Part model, mm, in its own coordinate system. A direction names the side the tool comes from. Round coordinates to 2 decimals unless told otherwise and drop trailing zeros. Loops run counter-clockwise (first coordinate to the right, second up) from the corner with the lowest first, then second, coordinate; pieces in that order, holes last. Notation, with made-up numbers: M 28.25,-10.75 L 47.25,-10.75 A33 cw 47.25,28.25 Z; hole C 23.5,-36.5 d3. An arc over 180 degrees is marked long. Put each result on its own line as item: value. Start each with the question number.
```python
from build123d import *

# Parameters (mm, degrees)
SALIENTE_EXTRUIR1_DEPTH      = 5
SALIENTE_EXTRUIR1_DEPTH_BACK = 5
CROQUIS1_W                   = 3
CROQUIS1_H                   = 75
SALIENTE_EXTRUIR3_DEPTH      = 7.5
SALIENTE_EXTRUIR3_DEPTH_BACK = 7.5
CROQUIS1_4_R                 = 3
CROQUIS1_4_R_2               = 1.5
CORTAR_EXTRUIR1_DEPTH        = 2.5
CORTAR_EXTRUIR1_DEPTH_BACK   = 2.5
CROQUIS1_5_R                 = 3
CORTAR_EXTRUIR2_DEPTH        = 10
CORTAR_EXTRUIR2_DEPTH_BACK   = 10
CROQUIS1_6_R                 = 1.5


with BuildPart() as part:
    # Croquis1 → Saliente-Extruir1 (new, two sides: drawn at the far end of the back side and taken through both)
    with BuildSketch(Plane.XY.offset(-SALIENTE_EXTRUIR1_DEPTH_BACK)):
        Rectangle(CROQUIS1_W, CROQUIS1_H)
    extrude(amount=SALIENTE_EXTRUIR1_DEPTH + SALIENTE_EXTRUIR1_DEPTH_BACK)

    # Croquis1_4 → Saliente-Extruir3 (add, two sides: drawn at the far end of the back side and taken through both)
    # profile 1 of 2: a face of its own
    with BuildSketch(Plane.XY.offset(-SALIENTE_EXTRUIR3_DEPTH_BACK)):
        with Locations((0, 37.5)):
            Circle(CROQUIS1_4_R)
        with Locations((0, 37.5)):
            Circle(CROQUIS1_4_R_2, mode=Mode.SUBTRACT)
    # profile 2 of 2: a face of its own
    with BuildSketch(Plane.XY.offset(-SALIENTE_EXTRUIR3_DEPTH_BACK)):
        with Locations((0, -37.5)):
            Circle(CROQUIS1_4_R)
        with Locations((0, -37.5)):
            Circle(CROQUIS1_4_R_2, mode=Mode.SUBTRACT)
    extrude(amount=SALIENTE_EXTRUIR3_DEPTH + SALIENTE_EXTRUIR3_DEPTH_BACK)

    # Croquis1_5 → Cortar-Extruir1 (cut, two sides: drawn at the far end of the back side and taken through both)
    with BuildSketch(Plane.XY.offset(-CORTAR_EXTRUIR1_DEPTH_BACK)):
        with Locations((0, 37.5)):
            Circle(CROQUIS1_5_R)
        with Locations((0, -37.5)):
            Circle(CROQUIS1_5_R)
    extrude(amount=CORTAR_EXTRUIR1_DEPTH + CORTAR_EXTRUIR1_DEPTH_BACK, mode=Mode.SUBTRACT)

    # Croquis1_6 → Cortar-Extruir2 (cut, two sides: drawn at the far end of the back side and taken through both)
    with BuildSketch(Plane.XY.offset(-CORTAR_EXTRUIR2_DEPTH_BACK)):
        with Locations((0, 37.5)):
            Circle(CROQUIS1_6_R)
        with Locations((0, -37.5)):
            Circle(CROQUIS1_6_R)
    extrude(amount=CORTAR_EXTRUIR2_DEPTH + CORTAR_EXTRUIR2_DEPTH_BACK, mode=Mode.SUBTRACT)

    # Croquis1_11 → Cortar-Revoluci_n2 (revolve, cut)
    with BuildSketch(Plane.XY):
        with BuildLine():
            ThreePointArc((-3, -37.5), (0, -40.5), (3, -37.5))
            Line((3, -37.5), (1.5, -37.5))
            ThreePointArc((1.5, -37.5), (0, -39), (-1.5, -37.5))
            Line((-1.5, -37.5), (-3, -37.5))
        make_face()
        with BuildLine():
            ThreePointArc((-1.5, -37.5), (0, -39), (1.5, -37.5))
            Line((1.5, -37.5), (-1.5, -37.5))
        make_face()
        with BuildLine():
            Line((-1.5, -37.5), (1.5, -37.5))
            ThreePointArc((1.5, -37.5), (0, -36), (-1.5, -37.5))
        make_face()
    revolve(axis=Axis((3, -37.5, 0), (-1, 0, 0)), mode=Mode.SUBTRACT)


solid = part.part
```
1. Wall check: L1, parallel to Y at x = 0, z = 3.95; L2, parallel to Y at x = 0, z = -5.45; L3, parallel to Z at x = 1.35, y = 35. Give the ranges that are in metal, low to high.
2. Cut at B-B, the plane z = -6. Give the cut face in (x, y).
3. Cut at D-D, the plane y = 37.5. Give the cut face in (x, z), and give its area (3 significant figures).
4. Cut at C-C, the plane x = 0. Give the number of separate pieces and of enclosed holes in the cut face, and give its area (3 significant figures).
5. Mould opens along X. For faces 6 (the cylindrical face through (0, 36, 5)), 7 (the flat face through (-1.5, 0, 0)), 8 (the flat face through (1, -36, -7.5)), 9 (the cylindrical face through (1.384, -40.162, -5.035)) say: released by +X, released by -X, zero draft, split by the parting line, or undercut.
6. Cut at A-A, the plane y = -37.5. Give the cut face in (x, z), and give its area (3 significant figures).
7. Which spindle directions (+Z, -Z, +X, -X, +Y, -Y) get a long thin tool onto all of the face, cutting with end or side? Do faces 1 (the flat face through (0, 0, -5)), 2 (the cylindrical face through (0, -34.5, 0)), 3 (the flat face through (1.5, 0, 0)), 4 (the flat face through (1, 39, 7.5)), 5 (the flat face through (0, 0, 5)). Say none if no direction does.
8. Drop flat-ended pins along their axis: pin 1 (8 mm diameter, centred on y = -8.5, z = -1, fed in from +X); pin 2 (8 mm diameter, centred on y = -16, z = 2.5, fed in from -X); pin 3 (3.5 mm diameter, centred on x = 0.5, y = 9, fed in from -Z). Give the stop position or say it passes through.
Results list:
1. L1: y = -40.5 to -39, -36 to 36, 39 to 40.5
1. L2: y = -40.5 to -39, -36 to -34.5, 34.5 to 36, 39 to 40.5
1. L3: z = -7.5 to -2.5, 2.5 to 7.5
2. outline: C 0,-37.5 d6; C 0,37.5 d6; hole C 0,-37.5 d3; hole C 0,37.5 d3
3. outline: M -3,-7.5 L -1.5,-7.5 L -1.5,-2.5 L -3,-2.5 Z; M -3,2.5 L -1.5,2.5 L -1.5,7.5 L -3,7.5 Z; M 1.5,-7.5 L 3,-7.5 L 3,-2.5 L 1.5,-2.5 Z; M 1.5,2.5 L 3,2.5 L 3,7.5 L 1.5,7.5 Z
3. area: 30.0 mm^2
4. separate pieces: 5
4. enclosed holes: 0
4. area: 750 mm^2
5. face 6: undercut
5. face 7: released by -X
5. face 8: zero draft
5. face 9: split by the parting line
6. outline: M -3,-7.5 L -1.5,-7.5 L -1.5,-2.6 A3 cw -1.66,-2.5 L -3,-2.5 Z; M -3,2.5 L -1.66,2.5 A3 cw -1.5,2.6 L -1.5,7.5 L -3,7.5 Z; M 1.5,-7.5 L 3,-7.5 L 3,-2.5 L 1.66,-2.5 A3 cw 1.5,-2.6 Z; M 1.5,2.6 A3 cw 1.66,2.5 L 3,2.5 L 3,7.5 L 1.5,7.5 Z
6. area: 30.0 mm^2
7. face 1: -Z, +X, -X
7. face 2: -Y
7. face 3: +Z, -Z, +X
7. face 4: +Z, +X, -X, +Y, -Y
7. face 5: +Z, +X, -X
8. pin 1: stops at x = 1.5
8. pin 2: stops at x = -1.5
8. pin 3: stops at z = -5
